The listing builds one solid part. Answer for the finished solid, in the listing's coordinates (mm). Face numbers are marked on the shaded views. A direction names the side the tool comes from. Give positions to 0.01 mm unless a question says otherwise; leave off trailing zeros. Write each loop counter-clockwise with the first axis right and the second up, starting at its lowest first coordinate (ties: lowest second). Pieces come first, ordered by that corner, then holes. Notation, with made-up numbers: (-21, -12) - (36, -12) arc R17 cw to (36, -8) - close; hole circle Ø3 at (31, -38). An arc over 180 degrees is marked (long way). Answer in a Markdown table with one row per item. Add a question column.
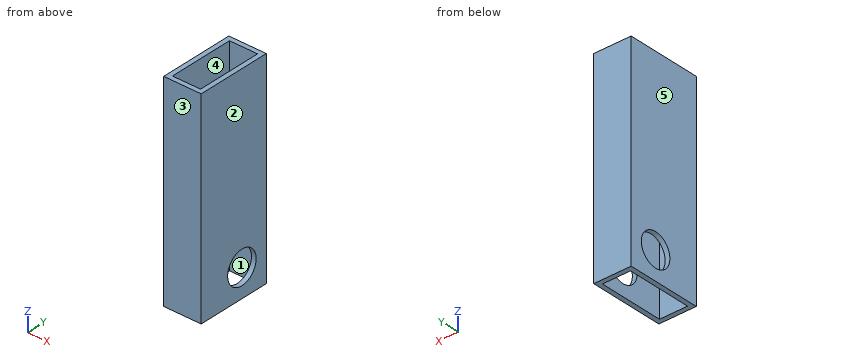
Autodesk Inventor part; units mm, degrees
ref_plane "YZ Plane" through (0, 0, 0) normal (1, 0, 0) x (0, 1, 0)
ref_plane "XZ Plane" through (0, 0, 0) normal (0, 1, 0) x (-1, 0, 0)
ref_plane "XY Plane" through (0, 0, 0) normal (0, 0, 1) x (1, 0, 0)
sketch "Sketch1" plane through (0, 0, 0) normal (0, 0, 1) x (1, 0, 0)
  line L0 (-12.7, 25.4) -> (12.7, 25.4)
  line L1 (12.7, 25.4) -> (12.7, -25.4)
  line L2 (12.7, -25.4) -> (-12.7, -25.4)
  line L3 (-12.7, -25.4) -> (-12.7, 25.4)
  line L4 (-12.7, 25.4) -> (12.7, -25.4) construction
  line L5 (12.7, 25.4) -> (-12.7, -25.4) construction
  line L6 (-9.525, -22.225) -> (9.525, -22.225)
  line L7 (9.525, -22.225) -> (9.525, 22.225)
  line L8 (9.525, 22.225) -> (-9.525, 22.225)
  line L9 (-9.525, 22.225) -> (-9.525, -22.225)
  line L10 (-9.525, -22.225) -> (9.525, 22.225) construction
  line L11 (9.525, -22.225) -> (-9.525, 22.225) construction
  point P0 (0, 0)
  dimension "d0" = 50.8
  dimension "d1" = 25.4
  dimension "d2" = 3.175
  dimension "d3" = 3.175
extrude "Extrusion1" add sketch "Sketch1" along normal blind 139.7
sketch "Sketch2" plane through (12.7, -25.4, 0) normal (1, 0, 0) x (0, 0, -1)
  circle A0 centre (-19.05, 31.75) radius 11.1125
  line L0 (0, 50.8) -> (-139.7, 50.8)
  point P0 (0, 25.4)
  dimension "d6" = 22.225
  dimension "d7" = 19.05
  dimension "d8" = 19.05
extrude "Extrusion2" cut sketch "Sketch2" against normal through all
equation "\"d3\" = d2"
properties part number "pivot block" material "Aluminum 6061"
1. A tool of negligible diameter and unlimited length cuts with its end or side. For the marked faces 4 and 5, from which of +Z, -Z, +X, -X, +Y, -Y can it reach the whole face along a straight path? Write none if from no direction.
2. Section D-D (z = 102) is taken. Give the vertices of the cut face in (x, y) (3 decimals).
3. The mould has two halves that part along X. Classify the marked faces 1, 2 and 3: +X half, -X half, draft (parallel to the pull), parting line (faces both ways), or undercut.
4. Given pin 1 Ø10 at (y, z) = (-0.5, 25.5) entering from +X, flat-ended and moving along its own axis, determine where the tip first touches the part or whether it passes through.
5. Section C-C (y = 6.35) is taken. Give the vertices of the cut face in (x, z) (1 decimal).
6. Section B-B (x = 6) is taken. Give the vertices of the cut face in (y, z) (3 decimals).
7. Straight lines are drawn through the part: L1, parallel to X at y = -5, z = 11.5 (3 decimals); L2, parallel to Y at x = -9, z = 78 (3 decimals); L3, parallel to Y at x = -11.3, z = 19.05. For each, find the intervals that lie inside material, in ascending order. Write a range as [from, to].
8. Section A-A (z = 19.05) is taken. Give the vertices of the cut face in (x, y) (1 decimal), and give its area (3 significant figures).
Geometry check:
| question | item | result |
|---|---|---|
| 1 | face 4 | +Z, -Z |
| 1 | face 5 | +Z, -Z, -X, +Y, -Y |
| 2 | outline | (-12.7, -25.4) - (12.7, -25.4) - (12.7, 25.4) - (-12.7, 25.4) - close; hole (-9.525, -22.225) - (9.525, -22.225) - (9.525, 22.225) - (-9.525, 22.225) - close |
| 3 | face 1 | undercut |
| 3 | face 2 | +X half |
| 3 | face 3 | draft |
| 4 | pin 1 | x = 12.7 |
| 5 | outline | (-12.7, 0) - (-9.5, 0) - (-9.5, 7.9) - (-12.7, 7.9) - close; (-12.7, 30.2) - (-9.5, 30.2) - (-9.5, 139.7) - (-12.7, 139.7) - close; (9.5, 0) - (12.7, 0) - (12.7, 7.9) - (9.5, 7.9) - close; (9.5, 30.2) - (12.7, 30.2) - (12.7, 139.7) - (9.5, 139.7) - close |
| 6 | outline | (-25.4, 0) - (-22.225, 0) - (-22.225, 139.7) - (-25.4, 139.7) - close; (22.225, 0) - (25.4, 0) - (25.4, 139.7) - (22.225, 139.7) - close |
| 7 | L1 | [-12.7, -9.525], [9.525, 12.7] |
| 7 | L2 | [-25.4, -22.225], [22.225, 25.4] |
| 7 | L3 | [-25.4, -4.76], [17.46, 25.4] |
| 8 | outline | (-12.7, -25.4) - (12.7, -25.4) - (12.7, -4.8) - (9.5, -4.8) - (9.5, -22.2) - (-9.5, -22.2) - (-9.5, -4.8) - (-12.7, -4.8) - close; (-12.7, 17.5) - (-9.5, 17.5) - (-9.5, 22.2) - (9.5, 22.2) - (9.5, 17.5) - (12.7, 17.5) - (12.7, 25.4) - (-12.7, 25.4) - close |
| 8 | area | 302 mm² |
